The model under review builds one solid part; all positions refer to its coordinate system, in mm. A direction names the side the tool comes from. Round coordinates to 2 decimals unless told otherwise and drop trailing zeros. Loops run counter-clockwise (first coordinate to the right, second up) from the corner with the lowest first, then second, coordinate; pieces in that order, holes last. Notation, with made-up numbers: (-25, 23.25) -> (24, 23.25) arc R18 cw to (24, 39.25) -> close; hole circle Ø6 at (40.25, 79.25). An arc over 180 degrees is marked (long way). Write each question's results on one line, items separated by ' | '. Start each with the question number.
Item 1: We need section A-A (y = 14). Give the boundary of the cut face in (x, z).
Item 2: For L1, parallel to Y at x = -98, z = -125; L2, parallel to Z at x = 154, y = 36; L3, parallel to X at y = 25, z = 5.5, list the stretches that pass through material, from the lowest coordinate up. Write a range as from..to.
Item 3: Clearance check with flat-ended pins moving along their axes: pin 1 Ø6.5 at (x, z) = (63.11, 117.11) entering from -Y; pin 2 Ø4 at (x, y) = (-29.5, 30.5) entering from -Z; pin 3 Ø16.5 at (y, z) = (40, -85.5) entering from -X; pin 4 Ø10 at (x, y) = (162.5, 8.5) entering from +Z. State where each tip first meets the part, or that it passes through.
Item 4: Tool access review of faces 3 (the flat face through (73.112, 43, 138)), 4 (the cylindrical face through (3.76, 18.66, -185.93)): name each direction out of +Z, -Z, +X, -X, +Y, -Y from which nothing blocks a thin tool from reaching the whole face with its end or side.
Item 5: Mouldability with a two-part tool opening along Z and no side actions: class faces 1 (the cylindrical face through (-1.43, 43.49, -190.93)), 2 (the flat face through (43, 50, -3)) as pulls with the +Z half, pulls with the -Z half, needs draft (parallel to the pull), parting line crosses it, or undercut.
from build123d import *

# Parameters (mm, degrees)
SKETCH1_R              = 205
BOSS_EXTRUDE1_DEPTH    = 50
SKETCH2_R              = 15.25
CUT_EXTRUDE1_DEPTH     = 15
M12_TAPPED_HOLE3_D     = 10.2
M12_TAPPED_HOLE3_DEPTH = 26.185610843
M12_TAPPED_HOLE3_TIP   = 3.064389157
SKETCH3_W              = 30
SKETCH3_H              = 60
CUT_EXTRUDE2_DEPTH     = 15
M6_TAPPED_HOLE3_D      = 5
M6_TAPPED_HOLE3_DEPTH  = 13.497848452
M6_TAPPED_HOLE3_TIP    = 1.502151548
M12_TAPPED_HOLE2_D     = 10.2
M12_TAPPED_HOLE2_DEPTH = 26.185610843
M12_TAPPED_HOLE2_TIP   = 3.064389157
SKETCH35_R             = 4
CUT_EXTRUDE4_DEPTH     = 51
SKETCH36_R             = 11
CUT_EXTRUDE5_DEPTH     = 13.2
SKETCH37_R             = 7
CUT_EXTRUDE6_DEPTH     = 37.8
FILLET1_R              = 0.5
M6_TAPPED_HOLE4_D      = 5
M6_TAPPED_HOLE4_DEPTH  = 13.497848452
M6_TAPPED_HOLE4_TIP    = 1.502151548
M6_TAPPED_HOLE5_D      = 5
M6_TAPPED_HOLE5_DEPTH  = 13.497848452
M6_TAPPED_HOLE5_TIP    = 1.502151548
SKETCH46_R             = 3
CUT_EXTRUDE7_DEPTH     = 15
M12_TAPPED_HOLE1_D     = 10.2
M12_TAPPED_HOLE1_DEPTH = 26.185610843
M12_TAPPED_HOLE1_TIP   = 3.064389157


with BuildPart() as part:
    # Sketch1 → Boss-Extrude1 (new body)
    with BuildSketch(Plane(origin=(0, 0, 0), x_dir=(1, 0, 0), z_dir=(0, 1, 0))):
        Circle(SKETCH1_R)
    extrude(amount=BOSS_EXTRUDE1_DEPTH)

    # Sketch2 → Cut-Extrude1 (cut)
    with BuildSketch(Plane(origin=(0, 50, 0), x_dir=(1, 0, 0), z_dir=(0, 1, 0))):
        with Locations((-42.327685627, 31.896492385)):
            Circle(SKETCH2_R)
        with Locations((60.971197017, -32.546169272)):
            Circle(SKETCH2_R)
        with BuildLine():
            Line((22.508129816, -48.531499254), (11.656226811, -97.298662399))
            ThreePointArc((11.656226811, -97.298662399), (-29.77179649, -62.488909666), (22.508129816, -48.531499254))
        make_face()
        with BuildLine():
            Line((2.66745507, 66.354666069), (48.721770829, 66.354666069))
            ThreePointArc((48.721770829, 66.354666069), (25.69461295, 15.854666069), (2.66745507, 66.354666069))
        make_face()
    extrude(amount=-CUT_EXTRUDE1_DEPTH, mode=Mode.SUBTRACT)

    # M12 Tapped Hole3
    with Locations(Plane(origin=(0, 50, 0), x_dir=(1, 0, 0), z_dir=(0, 1, 0))):
        with Locations((-0.014790744, 0.024833856)):
            Hole(M12_TAPPED_HOLE3_D / 2, depth=M12_TAPPED_HOLE3_DEPTH)
            with Locations((0, 0, -(M12_TAPPED_HOLE3_DEPTH + M12_TAPPED_HOLE3_TIP / 2))):  # 118° drill point
                Cone(0, M12_TAPPED_HOLE3_D / 2, M12_TAPPED_HOLE3_TIP, mode=Mode.SUBTRACT)

    # Sketch3 → Cut-Extrude2 (cut)
    with BuildSketch(Plane(origin=(0, 50, 0), x_dir=(1, 0, 0), z_dir=(0, 1, 0))):
        with Locations((58.112318667, -137.113872591)):
            Rectangle(SKETCH3_W, SKETCH3_H)
        Polygon((110.814391162, 111.220861865), (81.72598544, 58.743584377), (107.964624184, 44.199381516), (137.053029906, 96.676659004), align=None)
        with Locations((-100.327685627, 99.896492385)):
            Rectangle(SKETCH3_W, SKETCH3_H)
        with Locations((-57.887681333, -137.113872591)):
            Rectangle(SKETCH3_W, SKETCH3_H)
        Polygon((9.358321352, 167.458446261), (35.596960096, 152.9142434), (10.672314373, 107.948645684), (10.672314373, 99.896492385), (30.672314373, 99.896492385), (30.672314373, 69.896492385), (0.672314373, 69.896492385), (0.672314373, 129.896492385), (10.672314373, 129.896492385), (11.746380439, 131.834173793), (-5.185881509, 141.219807517), align=None)
    extrude(amount=-CUT_EXTRUDE2_DEPTH, mode=Mode.SUBTRACT)

    # M6 Tapped Hole3
    with Locations(Plane(origin=(0, 35, 0), x_dir=(1, 0, 0), z_dir=(0, 1, 0))):
        with Locations((123.458749371, 92.77851371), (104.06647889, 57.793662051), (-105.327685627, 119.896492385), (-105.327685627, 79.896492385), (-62.887681333, -117.113872591), (-62.887681333, -157.113872591), (63.112318667, -117.113872591), (63.112318667, -157.113872591), (13.256466646, 153.864165726), (20.672314373, 79.896492385)):
            Hole(M6_TAPPED_HOLE3_D / 2, depth=M6_TAPPED_HOLE3_DEPTH)
            with Locations((0, 0, -(M6_TAPPED_HOLE3_DEPTH + M6_TAPPED_HOLE3_TIP / 2))):  # 118° drill point
                Cone(0, M6_TAPPED_HOLE3_D / 2, M6_TAPPED_HOLE3_TIP, mode=Mode.SUBTRACT)

    # M12 Tapped Hole2
    with Locations(Plane(origin=(0, 50, 0), x_dir=(1, 0, 0), z_dir=(0, 1, 0))):
        with Locations((35.989041426, -60.006192032)):
            Hole(M12_TAPPED_HOLE2_D / 2, depth=M12_TAPPED_HOLE2_DEPTH)
            with Locations((0, 0, -(M12_TAPPED_HOLE2_DEPTH + M12_TAPPED_HOLE2_TIP / 2))):  # 118° drill point
                Cone(0, M12_TAPPED_HOLE2_D / 2, M12_TAPPED_HOLE2_TIP, mode=Mode.SUBTRACT)

    # Sketch35 → Cut-Extrude4 (cut, through all)
    with BuildSketch(Plane(origin=(0, 50, 0), x_dir=(1, 0, 0), z_dir=(0, 1, 0))):
        with Locations((-175.014790744, 0.024833856)):
            Circle(SKETCH35_R)
        with Locations((174.985209256, 0.024833856)):
            Circle(SKETCH35_R)
    extrude(amount=-CUT_EXTRUDE4_DEPTH, mode=Mode.SUBTRACT)

    # Sketch36 → Cut-Extrude5 (cut)
    with BuildSketch(Plane(origin=(0, 50, 0), x_dir=(1, 0, 0), z_dir=(0, 1, 0))):
        with Locations((0, 180.024833248)):
            Circle(SKETCH36_R)
        with Locations((155.906078905, -90.012416624)):
            Circle(SKETCH36_R)
        with Locations((-155.906078905, -90.012416624)):
            Circle(SKETCH36_R)
    extrude(amount=-CUT_EXTRUDE5_DEPTH, mode=Mode.SUBTRACT)

    # Sketch37 → Cut-Extrude6 (cut, through all)
    with BuildSketch(Plane(origin=(0, 36.8, 0), x_dir=(1, 0, 0), z_dir=(0, 1, 0))):
        with Locations((0, 180.024833248)):
            Circle(SKETCH37_R)
        with Locations((155.906078905, -90.012416624)):
            Circle(SKETCH37_R)
        with Locations((-155.906078905, -90.012416624)):
            Circle(SKETCH37_R)
    extrude(amount=-CUT_EXTRUDE6_DEPTH, mode=Mode.SUBTRACT)

    # Fillet1
    fillet1_edges = [part.edges().sort_by_distance(p)[0] for p in [
        (11.656226811, 42.5, 97.298662399),
        (22.508129816, 42.5, 48.531499254),
        (48.721770829, 42.5, -66.354666069),
        (2.66745507, 42.5, -66.354666069),
        (-85.327685627, 42.5, -129.896492385),
        (-85.327685627, 42.5, -69.896492385),
        (-115.327685627, 42.5, -69.896492385),
        (-115.327685627, 42.5, -129.896492385),
        (-205, 50, 0),
        (30.672314373, 42.5, -99.896492385),
        (30.672314373, 42.5, -69.896492385),
        (0.672314373, 42.5, -69.896492385),
        (0.672314373, 42.5, -129.896492385),
        (-5.185881509, 42.5, -141.219807517),
        (9.358321352, 42.5, -167.458446261),
        (35.596960096, 42.5, -152.9142434),
        (43.112318667, 42.5, 107.113872591),
        (73.112318667, 42.5, 107.113872591),
        (73.112318667, 42.5, 167.113872591),
        (43.112318667, 42.5, 167.113872591),
        (-42.887681333, 42.5, 107.113872591),
        (-42.887681333, 42.5, 167.113872591),
        (-72.887681333, 42.5, 167.113872591),
        (-72.887681333, 42.5, 107.113872591),
        (137.053029906, 42.5, -96.676659004),
        (107.964624184, 42.5, -44.199381516),
        (81.72598544, 42.5, -58.743584377),
        (110.814391162, 42.5, -111.220861865),
    ]]
    fillet(fillet1_edges, radius=FILLET1_R)

    # M6 Tapped Hole4
    with Locations(Plane(origin=(0, 35, 0), x_dir=(1, 0, 0), z_dir=(0, 1, 0))):
        with Locations((5.69461295, 46.354666069), (25.69461295, 26.354666069), (45.69461295, 46.354666069)):
            Hole(M6_TAPPED_HOLE4_D / 2, depth=M6_TAPPED_HOLE4_DEPTH)
            with Locations((0, 0, -(M6_TAPPED_HOLE4_DEPTH + M6_TAPPED_HOLE4_TIP / 2))):  # 118° drill point
                Cone(0, M6_TAPPED_HOLE4_D / 2, M6_TAPPED_HOLE4_TIP, mode=Mode.SUBTRACT)

    # M6 Tapped Hole5
    with Locations(Plane(origin=(0, 35, 0), x_dir=(1, 0, 0), z_dir=(0, 1, 0))):
        with Locations((-19.522489502, -64.769634607), (4.344237984, -49.591383089), (-4.344237984, -88.636362093)):
            Hole(M6_TAPPED_HOLE5_D / 2, depth=M6_TAPPED_HOLE5_DEPTH)
            with Locations((0, 0, -(M6_TAPPED_HOLE5_DEPTH + M6_TAPPED_HOLE5_TIP / 2))):  # 118° drill point
                Cone(0, M6_TAPPED_HOLE5_D / 2, M6_TAPPED_HOLE5_TIP, mode=Mode.SUBTRACT)

    # Sketch46 → Cut-Extrude7 (cut)
    with BuildSketch(Plane(origin=(0, 35, 0), x_dir=(1, 0, 0), z_dir=(0, 1, 0))):
        with Locations((-12.657243637, -77.163356022)):
            Circle(SKETCH46_R)
        with Locations((12.657243637, -61.06438916)):
            Circle(SKETCH46_R)
        with Locations((15.088011232, 35.748064351)):
            Circle(SKETCH46_R)
        with Locations((36.301214668, 56.961267787)):
            Circle(SKETCH46_R)
    extrude(amount=-CUT_EXTRUDE7_DEPTH, mode=Mode.SUBTRACT)

    # M12 Tapped Hole1
    with Locations(Plane(origin=(0, 35, 0), x_dir=(1, 0, 0), z_dir=(0, 1, 0))):
        with Locations((-42.327685627, 31.896492385), (60.971197017, -32.546169272)):
            Hole(M12_TAPPED_HOLE1_D / 2, depth=M12_TAPPED_HOLE1_DEPTH)
            with Locations((0, 0, -(M12_TAPPED_HOLE1_DEPTH + M12_TAPPED_HOLE1_TIP / 2))):  # 118° drill point
                Cone(0, M12_TAPPED_HOLE1_D / 2, M12_TAPPED_HOLE1_TIP, mode=Mode.SUBTRACT)


solid = part.part
Here are the results:
1) outline: circle Ø410 at (0, 0); hole circle Ø8 at (-175.01, -0.02); hole circle Ø14 at (-155.91, 90.01); hole circle Ø10.2 at (-42.33, -31.9); hole circle Ø14 at (0, -180.02); hole circle Ø10.2 at (60.97, 32.55); hole circle Ø14 at (155.91, 90.01); hole circle Ø8 at (174.99, -0.02)
2) L1: y = 0..35 | L2: z = -135.31..83.28, 96.75..135.31 | L3: x = -204.93..204.93
3) pin 1: stops at y = 0 | pin 2: stops at z = -203.15 | pin 3: stops at x = -189.89 | pin 4: stops at z = 131.22
4) face 3: +Y | face 4: +Y, -Y
5) face 1: undercut | face 2: needs draft
